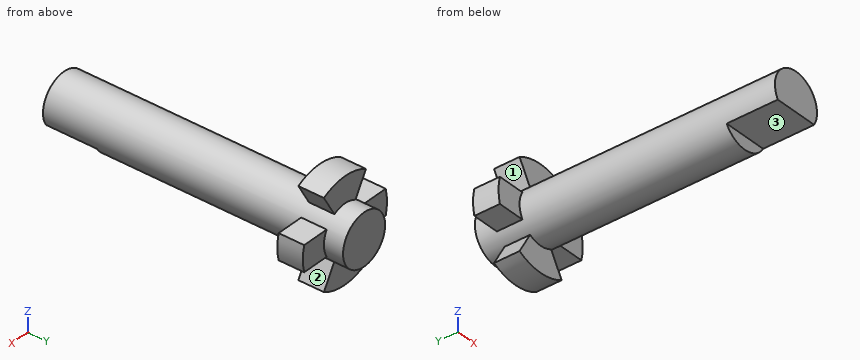
from build123d import *

# Parameters (mm, degrees)
SKETCH1_R           = 4
BOSS_EXTRUDE1_DEPTH = 47
BOSS_EXTRUDE2_DEPTH = 2
CUT_EXTRUDE1_DEPTH  = 8


with BuildPart() as part:
    # Sketch1 → Boss-Extrude1 (new body)
    with BuildSketch(Plane(origin=(0, 0, 0), x_dir=(1, 0, 0), z_dir=(0, 1, 0))):
        with Locations(Location((0, 0, 0), (0, 0, 270))):
            Circle(SKETCH1_R)
    extrude(amount=BOSS_EXTRUDE1_DEPTH)

    # Sketch2 → Boss-Extrude2 (add, symmetric)
    with BuildSketch(Plane(origin=(0, 42, 0), x_dir=(1, 0, 0), z_dir=(0, 1, 0))):
        with BuildLine():
            Line((-4, 6.92820323), (-2, 3.464101615))
            ThreePointArc((-2, 3.464101615), (0, 4), (2, 3.464101615))
            Line((2, 3.464101615), (4, 6.92820323))
            ThreePointArc((4, 6.92820323), (0, 8), (-4, 6.92820323))
        make_face()
        with BuildLine():
            Line((-7.745966692, 2), (-3.464101615, 2))
            ThreePointArc((-3.464101615, 2), (-4, 0), (-3.464101615, -2))
            Line((-3.464101615, -2), (-7.745966692, -2))
            ThreePointArc((-7.745966692, -2), (-8, 0), (-7.745966692, 2))
        make_face()
        with BuildLine():
            Line((7.745966692, 2), (3.464101615, 2))
            ThreePointArc((3.464101615, 2), (4, 0), (3.464101615, -2))
            Line((3.464101615, -2), (7.745966692, -2))
            ThreePointArc((7.745966692, -2), (8, 0), (7.745966692, 2))
        make_face()
        with BuildLine():
            Line((4, -6.92820323), (2, -3.464101615))
            ThreePointArc((2, -3.464101615), (0, -4), (-2, -3.464101615))
            Line((-2, -3.464101615), (-4, -6.92820323))
            ThreePointArc((-4, -6.92820323), (0, -8), (4, -6.92820323))
        make_face()
    extrude(amount=BOSS_EXTRUDE2_DEPTH, both=True)

    # Sketch3 → Cut-Extrude1 (cut)
    with BuildSketch(Plane.XZ):
        with BuildLine():
            Line((-3.464101615, -2), (3.464101615, -2))
            ThreePointArc((3.464101615, -2), (0, -4), (-3.464101615, -2))
        make_face()
    extrude(amount=-CUT_EXTRUDE1_DEPTH, mode=Mode.SUBTRACT)


solid = part.part
Verification items for the finished model (mm, model axes). Face numbers are marked on the shaded views. A direction names the side the tool comes from. Round coordinates to 2 decimals unless told otherwise and drop trailing zeros. Loops run counter-clockwise (first coordinate to the right, second up) from the corner with the lowest first, then second, coordinate; pieces in that order, holes last. Notation, with made-up numbers: (24.25, -11.75) - (58.25, -11.75) arc R19 cw to (58.25, 6.25) - close; hole circle Ø1 at (29, 13.25). An arc over 180 degrees is marked (long way). Answer in a Markdown table with one row per item. Add a question column.
Q1. Gauge pin test, flat ends, axial feed: pin 1 (2 mm diameter, centred on y = 32, z = -1.5, fed in from +X); pin 2 (2 mm diameter, centred on x = 5.5, y = 42.5, fed in from +Z); pin 3 (7.5 mm diameter, centred on x = 1.5, y = 5, fed in from -Z); pin 4 (1.5 mm diameter, centred on x = 4, z = -3.5, fed in from -Y). Record the tip position at first contact, or that the pin passes through.
Q2. Section check A-A on x = 0. Enter the section's corners in (y, z).
Q3. Section check D-D on x = -4.5. Enter the section's corners in (y, z), plus the area to 3 significant figures.
Q4. Tool access check on the marked faces 1, 2 and 3. Record the directions out of +Z, -Z, +X, -X, +Y, -Y that give a thin tool (end or side, any length) a straight path to the whole face; none if there is none.
Q5. Section check B-B on z = 0. Enter the section's corners in (x, y).
Q6. Material ranges on line 1 (Z direction, x = 0.25, y = 3); line 2 (Z direction, x = 0.25, y = 45.5); line 3 (Y direction, x = 0.25, z = 5.75), recorded low to high.
Q7. Section check C-C on y = 6. Enter the section's corners in (x, z).
Found:
| question | item | result |
|---|---|---|
| 1 | pin 1 | stops at x = 3.97 |
| 1 | pin 2 | stops at z = 2 |
| 1 | pin 3 | stops at z = -4 |
| 1 | pin 4 | passes through |
| 2 | outline | (0, -2) - (8, -2) - (8, -4) - (40, -4) - (40, -8) - (44, -8) - (44, -4) - (47, -4) - (47, 4) - (44, 4) - (44, 8) - (40, 8) - (40, 4) - (0, 4) - close |
| 3 | outline | (40, -2) - (44, -2) - (44, 2) - (40, 2) - close |
| 3 | area | 16.0 mm² |
| 4 | face 1 | -X, +Y, -Y |
| 4 | face 2 | +X, +Y, -Y |
| 4 | face 3 | -Z, +X, -X, -Y |
| 5 | outline | (-8, 40) - (-4, 40) - (-4, 0) - (4, 0) - (4, 40) - (8, 40) - (8, 44) - (4, 44) - (4, 47) - (-4, 47) - (-4, 44) - (-8, 44) - close |
| 6 | line 1 | z = -2 to 3.99 |
| 6 | line 2 | z = -3.99 to 3.99 |
| 6 | line 3 | y = 40 to 44 |
| 7 | outline | (-3.46, -2) - (3.46, -2) arc R4 ccw (long way) to start |
